Input: dimensioned drawing with shaded views. Units: mm. Origin: part minimum x, y, z. Give positions to 0.01 mm unless a question says otherwise; leave off trailing zeros. Loops run counter-clockwise (first coordinate to the right, second up) from the corner with the lowest first, then second, coordinate; pieces in that order, holes last.
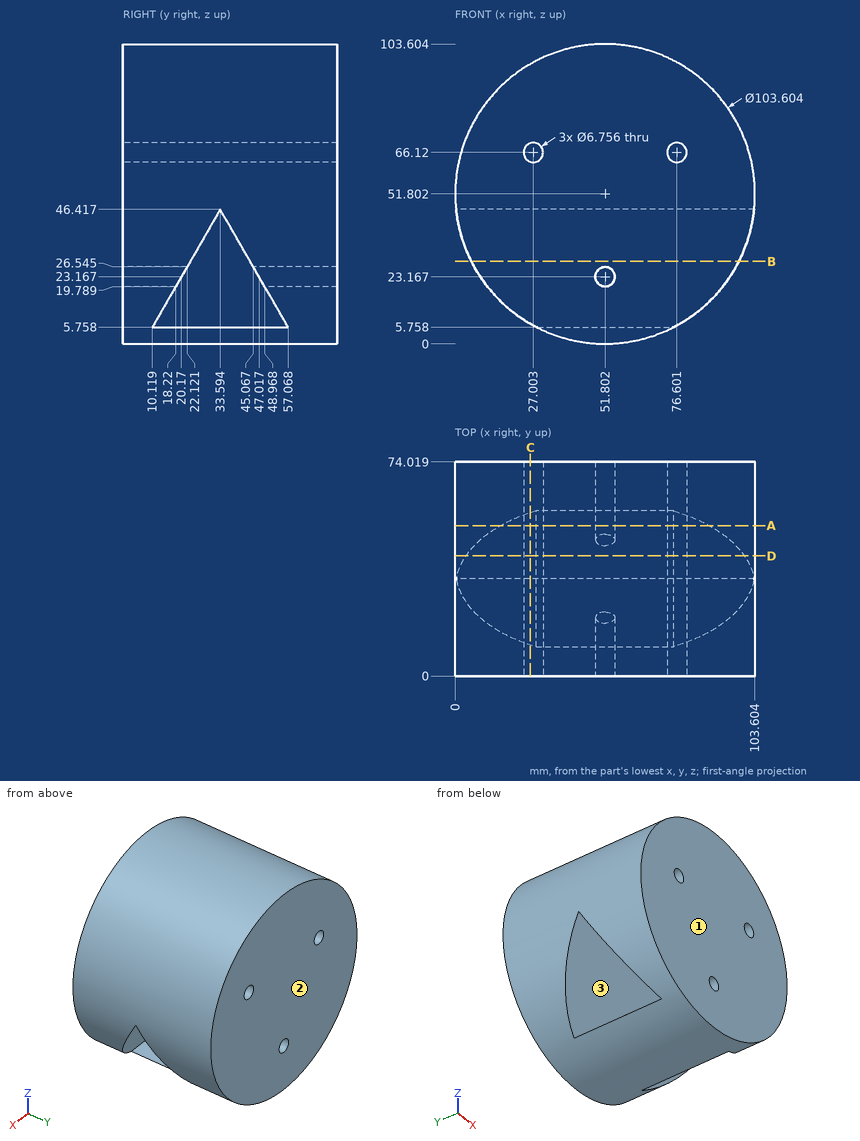
(1) Section B-B, the plane z = 28.5. Return the cut outline in (x, y).
A:
outline: (5.54, 0) - (98.07, 0) - (98.07, 23.25) - (5.54, 23.25) - close; (5.54, 43.94) - (98.07, 43.94) - (98.07, 74.02) - (5.54, 74.02) - close
(2) Mould query, pull axis Y, two halves, no side actions, for the marked faces 1, 2 and 3. Classes: pulls with the +Y half, pulls with the -Y half, needs draft (parallel to the pull), parting line crosses it, or undercut.
A:
face 1: pulls with the -Y half
face 2: pulls with the +Y half
face 3: undercut
(3) Section A-A, the plane y = 52. Return the cut outline in (x, z) (1 decimal).
A:
outline: (15.8, 14.5) - (87.8, 14.5) arc R51.8 ccw (long way) to start; (28.1, 5.8) arc R51.8 ccw to (75.5, 5.8) - close; hole circle Ø6.8 at (27, 66.1); hole circle Ø6.8 at (51.8, 23.2); hole circle Ø6.8 at (76.6, 66.1)
(4) Section C-C, the plane x = 26. Return the cut outline in (y, z) (1 decimal).
A:
outline: (0, 6.9) - (10.8, 6.9) - (33.6, 46.4) - (56.4, 6.9) - (74, 6.9) - (74, 62.9) - (0, 62.9) - close; (0, 69.3) - (74, 69.3) - (74, 96.7) - (0, 96.7) - close
(5) First-contact query: pin 1 (6 mm diameter, centred on x = 44.5, y = 26, fed in from -Z); pin 2 (5.5 mm diameter, centred on x = 76.6, z = 66.12, fed in from +Y); pin 3 (23.5 mm diameter, centred on x = 50, y = 37.5, fed in from +Z); pin 4 (2 mm diameter, centred on x = 59.5, y = 56, fed in from -Z) (1 decimal). Flat tips, straight axial feed; report the tip coordinate or a pass-through.
A:
pin 1: stops at z = 0.18
pin 2: passes through
pin 3: stops at z = 103.6
pin 4: stops at z = 0.4
(6) Ray query, line 1 along X through (y, z) = (64.5, 63.5) (1 decimal); line 2 along Z through (x, y) = (71, 12) (1 decimal); line 3 along Z through (x, y) = (45.5, 30) (1 decimal). Return the intervals inside material, ascending.
A:
line 1: x = 1.3 to 24.9, 29.1 to 74.5, 78.7 to 102.3
line 2: z = 3.7 to 5.8, 9 to 99.9
line 3: z = 0.4 to 5.8, 40.2 to 103.2
(7) Section D-D, the plane y = 41.5. Return the cut outline in (x, z) (1 decimal).
A:
outline: (3.6, 32.7) - (100, 32.7) arc R51.8 ccw (long way) to start; (28.1, 5.8) arc R51.8 ccw to (75.5, 5.8) - close; hole circle Ø6.8 at (27, 66.1); hole circle Ø6.8 at (76.6, 66.1)
